Can you work these out from the model? Positions are in its coordinate system, mm. Face numbers are marked on the shaded views. A direction names the side the tool comes from. Give positions to 0.01 mm unless a question says otherwise; leave off trailing zeros. Write each loop counter-clockwise with the first axis right and the second up, starting at its lowest first coordinate (ties: lowest second). Pieces come first, ordered by that corner, then holes. Notation, with made-up numbers: (60, 74) - (113, 74) arc R36 cw to (113, 108) - close; hole circle Ø9 at (-7.75, 27). An arc over 180 degrees is marked (long way). Use a Markdown table: item, result. Add a question column.
```python
from build123d import *

# Parameters (mm, degrees)
BOSS_EXTRUDE1_DEPTH     = 40
SKETCH2_W               = 35.5
SKETCH2_H               = 25
CUT_EXTRUDE1_DEPTH      = 40
CUT_EXTRUDE2_DEPTH      = 67.671301922
CUT_EXTRUDE2_DEPTH_BACK = 67.671301922
SKETCH3_R               = 1.25
FILLET2_R               = 5
CHAMFER1_SIZE           = 5
SKETCH4_W               = 17
SKETCH4_H               = 25
SKETCH4_W_2             = 10
CUT_EXTRUDE3_DEPTH      = 30
FILLET3_R               = 12


with BuildPart() as part:
    # Sketch1 → Boss-Extrude1 (new body)
    with BuildSketch(Plane.XY):
        Polygon((-14.25, -20), (21.25, -20), (21.25, -35), (34.25, -35), (34.25, 0), (-34.25, 0), (-34.25, -35), (-14.25, -35), align=None)
        Polygon((-34.25, -16), (-34.25, 0), (-34.25, 8), (-40.25, 8), (-40.25, -8), align=None)
        Polygon((34.25, 8), (34.25, 0), (34.25, -16), (40.25, -8), (40.25, 8), align=None)
    extrude(amount=BOSS_EXTRUDE1_DEPTH)

    # Sketch2 → Cut-Extrude1 (cut)
    with BuildSketch(Plane(origin=(0, 0, 0), x_dir=(1, 0, 0), z_dir=(0, 1, 0))):
        with Locations((3.5, -22.5)):
            Rectangle(SKETCH2_W, SKETCH2_H)
    extrude(amount=-CUT_EXTRUDE1_DEPTH, mode=Mode.SUBTRACT)

    # Sketch3 → Cut-Extrude2 (cut, two sides: drawn at the far end of the back side and taken through both)
    with BuildSketch(Plane(origin=(0, 0, 0), x_dir=(0, 0, -1), z_dir=(1, 0, 0)).offset(-CUT_EXTRUDE2_DEPTH_BACK)):
        with Locations((-35, 4)):
            Circle(SKETCH3_R)
        with Locations((-5, 4)):
            Circle(SKETCH3_R)
        with Locations((-20, 4)):
            Circle(SKETCH3_R)
    extrude(amount=CUT_EXTRUDE2_DEPTH + CUT_EXTRUDE2_DEPTH_BACK, mode=Mode.SUBTRACT)

    # Fillet2
    fillet2_edges = [part.edges().sort_by_distance(p)[0] for p in [
        (-37.25, 8, 0),
        (37.25, 8, 0),
        (37.25, 8, 40),
        (-34.25, -16, 20),
        (-40.25, -8, 20),
        (40.25, -8, 20),
        (34.25, -16, 20),
        (-37.25, 8, 40),
    ]]
    fillet(fillet2_edges, radius=FILLET2_R)

    # Chamfer1
    chamfer1_edges = [part.edges().sort_by_distance(p)[0] for p in [
        (21.25, -27.5, 0),
    ]]
    chamfer(chamfer1_edges, length=CHAMFER1_SIZE)

    # Sketch4 → Cut-Extrude3 (cut)
    with BuildSketch(Plane(origin=(0, 0, 0), x_dir=(1, 0, 0), z_dir=(0, 1, 0))):
        with Locations((-22.75, -22.5)):
            Rectangle(SKETCH4_W, SKETCH4_H)
        with Locations((26.25, -22.5)):
            Rectangle(SKETCH4_W_2, SKETCH4_H)
    extrude(amount=-CUT_EXTRUDE3_DEPTH, mode=Mode.SUBTRACT)

    # Fillet3
    # the kernel refuses this fillet: 12 mm, written as the material it adds along each edge
    with BuildSketch(Plane(origin=(-31.25, -30, 10), x_dir=(0, 1, 0), z_dir=(0, 0, 1))) as fillet3_piece_1_section:
        with BuildLine():
            CenterArc((FILLET3_R, -FILLET3_R), FILLET3_R, 90, 90)
            Line((0, -FILLET3_R), (0, 0))
            Line((0, 0), (FILLET3_R, 0))
        make_face()
    fillet3_piece_1 = extrude(amount=55, mode=Mode.PRIVATE)
    fillet3_piece_1 = split(fillet3_piece_1, bisect_by=Plane(origin=(-31.25, -30, 40), z_dir=(0, 0, -1)), keep=Keep.TOP, mode=Mode.PRIVATE)
    add(fillet3_piece_1)
    with BuildSketch(Plane(origin=(31.25, -30, 10), x_dir=(0, 1, 0), z_dir=(0, 0, 1))) as fillet3_piece_2_section:
        with BuildLine():
            CenterArc((11.832159566, 12), FILLET3_R, 189.594068227, 80.405931773)
            Line((0, 10), (0, 0))
            Line((0, 0), (11.832159566, 0))
        make_face()
    fillet3_piece_2 = extrude(amount=54.580398916, mode=Mode.PRIVATE)
    fillet3_piece_2 = split(fillet3_piece_2, bisect_by=Plane(origin=(31.25, -30, 40), z_dir=(0, 0, -1)), keep=Keep.TOP, mode=Mode.PRIVATE)
    add(fillet3_piece_2)
    # the kernel refuses this fillet: 12 mm, written as the material it takes off along each edge
    with BuildSketch(Plane(origin=(-34.25, -35, -30), x_dir=(1, 0, 0), z_dir=(0, 0, 1)), Plane(origin=(34.25, -35, -30), x_dir=(0, 1, 0), z_dir=(0, 0, 1))) as fillet3_2_piece_1:
        with BuildLine():
            CenterArc((FILLET3_R, FILLET3_R), FILLET3_R, 180, 90)
            Line((0, FILLET3_R), (0, 0))
            Line((0, 0), (FILLET3_R, 0))
        make_face()
    extrude(amount=100, mode=Mode.SUBTRACT)


solid = part.part
```
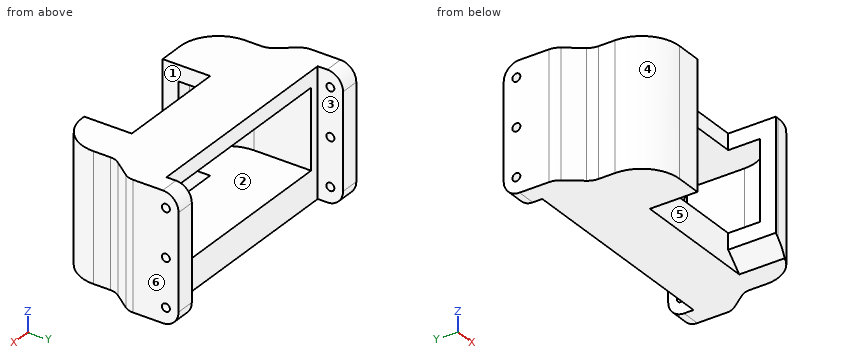
Q1. If I drill on probe 1 along Z at (x, y) = (-13, -17.5); probe 2 along Z at (x, y) = (-38.45, 4); probe 3 along X at (y, z) = (4, 27), over which ranges is the centre line in solid material (lowest first)? Write a range as [from, to].
Q2. I'm going to push flat-ended pins straight in: P1, Ø1.6, axis at y = -20.5, z = 21, coming from the -X side; P2, Ø2.5, axis at x = 9, z = 38, coming from the -Y side; P3, Ø2, axis at y = 4, z = 35, coming from the +X side; P4, Ø7.5, axis at y = -28.5, z = 11, coming from the +X side. Where does each tip first touch, or does it pass through?
Q3. Suppose I cut it at C-C (y = -1.5). Please give me the cut outline in (x, z).
Q4. On a 3-axis mill with a long thin cutter (end or side, diameter ignored), from which of +Z, -Z, +X, -X, +Y, -Y can I reach the whole of each face in a straight line? I mean the marked faces 1, 2 and 3. Say none if no direction works.
Q5. Suppose I cut it at B-B (x = 2). Please give me the cut outline in (y, z).
Q6. Suppose I cut it at A-A (z = 30). Please give me the cut outline in (x, y), and give its area (3 significant figures).
Q7. If we mould it in two halves opening along X, with no side actions, what happens to the marked faces 4, 5 and 6? For each: released by +X, released by -X, zero draft, split by the parting line, or undercut.
Q8. Suppose I cut it at D-D (y = -25). Please give me the cut outline in (x, z), and give its area (3 significant figures).
Derived:
| question | item | result |
|---|---|---|
| 1 | probe 1 | [0, 10], [35, 40] |
| 1 | probe 2 | [0.1, 3.75], [6.25, 18.75], [21.25, 33.75], [36.25, 39.9] |
| 1 | probe 3 | [-40.25, -34.25], [34.25, 40.25] |
| 2 | P1 | x = -34.25 |
| 2 | P2 | y = -20 |
| 2 | P3 | through |
| 2 | P4 | x = 34.12 |
| 3 | outline | (-40.25, 0) - (40.25, 0) - (40.25, 40) - (-40.25, 40) - close; hole (-31.25, 10) - (31.25, 10) - (31.25, 35) - (-31.25, 35) - close |
| 4 | face 1 | +Z, -Z, -Y |
| 4 | face 2 | +Y |
| 4 | face 3 | +Z, -Z, +Y |
| 5 | outline | (-20, 0) - (0, 0) - (0, 10) - (-20, 10) - close; (-20, 35) - (0, 35) - (0, 40) - (-20, 40) - close |
| 6 | outline | (-40.25, -6.33) arc R5 ccw to (-39.25, -9.33) - (-35.25, -14.67) arc R5 cw to (-34.25, -17.67) - (-34.25, -23) arc R12 ccw to (-22.25, -35) - (-14.25, -35) - (-14.25, -30) - (-19.25, -30) arc R12 cw to (-31.25, -18) - (-31.25, 0) - (-34.25, 0) - (-34.25, 8) - (-40.25, 8) - close; (21.25, -35) - (22.25, -35) arc R12 ccw to (34.25, -23) - (34.25, -17.67) arc R5 cw to (35.25, -14.67) - (39.25, -9.33) arc R5 ccw to (40.25, -6.33) - (40.25, 8) - (34.25, 8) - (34.25, 0) - (31.25, 0) - (31.25, -18.17) arc R12 cw to (21.25, -30) - close |
| 6 | area | 583 mm² |
| 7 | face 4 | released by -X |
| 7 | face 5 | undercut |
| 7 | face 6 | released by +X |
| 8 | outline | (-34.08, 0) - (-14.25, 0) - (-14.25, 10) - (-29, 10) - (-29, 35) - (-14.25, 35) - (-14.25, 40) - (-34.08, 40) - close; (21.25, 5) - (26.25, 0) - (34.08, 0) - (34.08, 40) - (21.25, 40) - (21.25, 35) - (29.12, 35) - (29.12, 10) - (21.25, 10) - close |
| 8 | area | 729 mm² |
